Print and shaded views of the part. All mm, measured from the part's lowest x, y and z. A direction names the side the tool comes from. Give positions to 0.01 mm unless a question says otherwise; leave off trailing zeros. Loops run counter-clockwise (first coordinate to the right, second up) from the corner with the lowest first, then second, coordinate; pieces in that order, holes last. Notation, with made-up numbers: (28.25, 51) - (56.25, 51) arc R25 ccw to (56.25, 73) - close; hole circle Ø5 at (-32.5, 0.25). An arc over 180 degrees is marked (long way). Return JSON: item names as keys, results as strings.
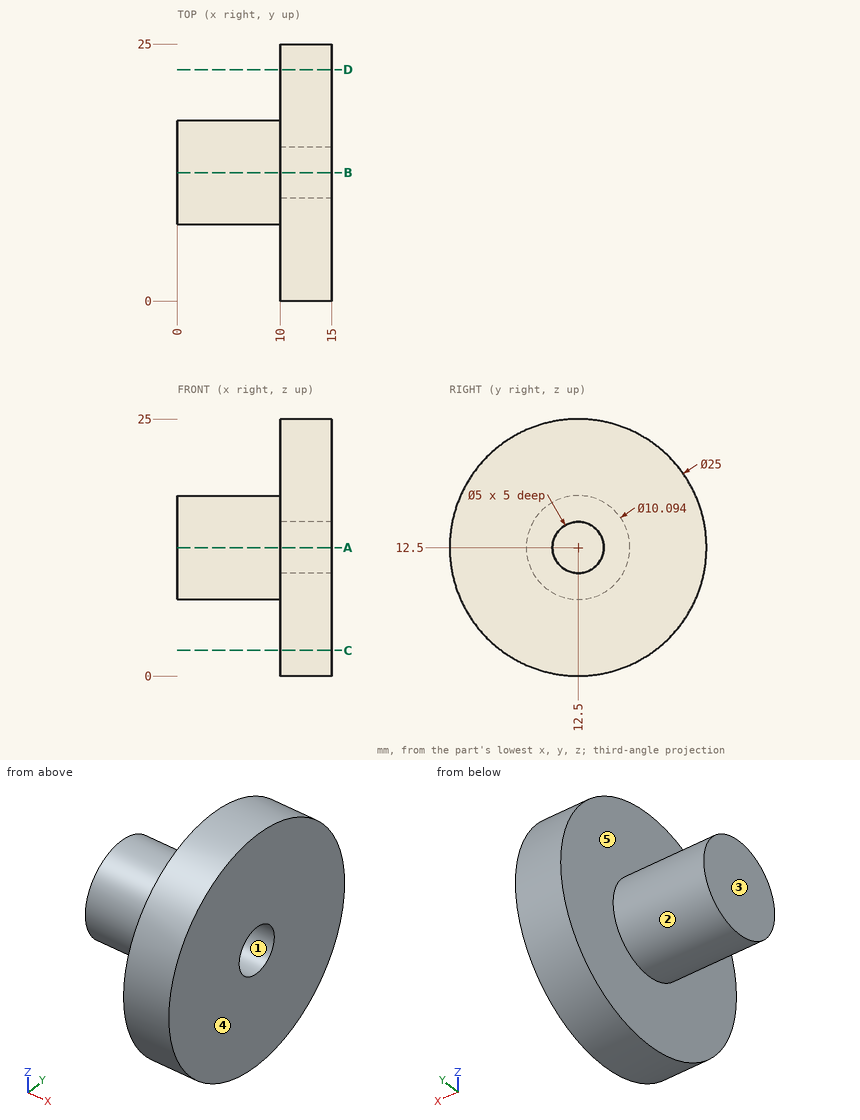
1. Cut at A-A, the plane z = 12.5. Write the cut outline in (x, y), plus the area to 3 significant figures.
Values follow:
{"outline": "(0, 7.45) - (10, 7.45) - (10, 0) - (15, 0) - (15, 10) - (10, 10) - (10, 15) - (15, 15) - (15, 25) - (10, 25) - (10, 17.55) - (0, 17.55) - close", "area": "201 mm²"}
2. Drill centre lines: probe 1 along Z at (x, y) = (12.4, 12.5); probe 2 along Z at (x, y) = (12.25, 13.5); probe 3 along X at (y, z) = (19.75, 18.25). Where is each one in solid material? Low to high.
Values follow:
{"probe 1": "z = 0 to 10, 15 to 25", "probe 2": "z = 0.04 to 10.21, 14.79 to 24.96", "probe 3": "x = 10 to 15"}
3. Drop flat-ended pins along their axis: P1, Ø6, axis at y = 20, z = 8, coming from the -X side; P2, Ø1, axis at x = 5, y = 8, coming from the -Z side; P3, Ø8, axis at x = 5.5, z = 10, coming from the +Y side. Give the stop position or say it passes through.
Values follow:
{"P1": "stops at x = 10", "P2": "stops at z = 9.42", "P3": "stops at y = 17.55"}
4. Cut at C-C, the plane z = 2.5. Write the cut outline in (x, y), plus the area to 3 significant figures.
Values follow:
{"outline": "(10, 5) - (15, 5) - (15, 20) - (10, 20) - close", "area": "75.0 mm²"}
5. Which spindle directions (+Z, -Z, +X, -X, +Y, -Y) get a long thin tool onto all of the face, cutting with end or side? Do the marked faces 4 and 5. Say none if no direction does.
Values follow:
{"face 4": "+Z, -Z, +X, +Y, -Y", "face 5": "-X"}
6. Pull direction Y, two halves, no side cores. Call the marked faces 1, 2 and 3: +Y half, -Y half, draft (parallel to the pull), parting line (faces both ways), or undercut.
Values follow:
{"face 1": "undercut", "face 2": "parting line", "face 3": "draft"}
